Could you check a few things on this model? Use its own coordinates, in mm. Face numbers are marked on the shaded views. A direction names the side the tool comes from. Give positions to 0.01 mm unless a question says otherwise; leave off trailing zeros. Write each loop counter-clockwise with the first axis right and the second up, starting at its lowest first coordinate (ties: lowest second). Pieces come first, ordered by that corner, then holes. Notation, with made-up numbers: M -38.75,-16.75 L -8.75,-16.75 A15 cw -8.75,1.25 Z; hole C -14,89.5 d2. An arc over 180 degrees is marked long. Answer as a JSON object with one key per item and string values. Group by question number.
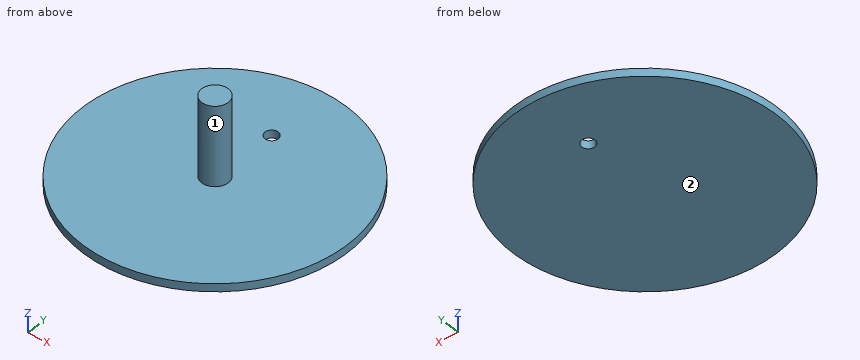
```python
from build123d import *

# Parameters (mm, degrees)
SKETCH_1_R          = 50
EXTRUDE_1_DEPTH     = 3
SKETCH_2_R          = 5
EXTRUDE_2_DEPTH     = 30
SKETCH_3_R          = 2.5
CUT_EXTRUDE_1_DEPTH = 77.811457479


with BuildPart() as part:
    # Эскиз1 → Бобышка-Вытянуть1 (new body)
    with BuildSketch(Plane.XY):
        Circle(SKETCH_1_R)
    extrude(amount=EXTRUDE_1_DEPTH)

    # Эскиз2 → Бобышка-Вытянуть2 (add)
    with BuildSketch(Plane.XY.offset(3)):
        Circle(SKETCH_2_R)
    extrude(amount=EXTRUDE_2_DEPTH)

    # Эскиз3 → Вырез-Вытянуть1 (cut, through all)
    with BuildSketch(Plane.XY.offset(3)):
        with Locations((0, 25)):
            Circle(SKETCH_3_R)
    extrude(amount=-CUT_EXTRUDE_1_DEPTH, mode=Mode.SUBTRACT)


solid = part.part
```
1) Please list where these lines run through material, in increasing order: line 1 along Y through (x, z) = (0, 2); line 2 along Z through (x, y) = (-18.5, -9.5); line 3 along X through (y, z) = (-4, 21.5). Write a range as from..to.
2) I'm going to push flat-ended pins straight in: pin 1 (10 mm diameter, centred on x = 39.5, y = 3.5, fed in from +Z); pin 2 (3 mm diameter, centred on x = 0, y = 25, fed in from -Z); pin 3 (1 mm diameter, centred on x = -19, y = 22, fed in from -Z); pin 4 (4 mm diameter, centred on x = 2, z = 11, fed in from -Y). Where does each tip first touch, or does it pass through?
3) If we section it at A-A, the plane x = 0: List the corners of the cut face in (y, z) for me, plus the area to 3 significant figures.
4) If we section it at D-D, the plane z = 5.5: List the corners of the cut face in (x, y) for me, plus the area to 3 significant figures.
5) For the marked faces 1 and 2, which set-ups out of +Z, -Z, +X, -X, +Y, -Y let a thin tool reach every point of the face, with its end or its side?
6) If we section it at C-C, the plane y = 0: List the corners of the cut face in (x, z) for me.
7) If we section it at B-B, the plane y = 25: List the corners of the cut face in (x, z) for me, plus the area to 3 significant figures.
Taken from the geometry:
{
 "1": {"line 1": "-50..22.5, 27.5..50", "line 2": "0..3", "line 3": "-3..3"},
 "2": {"pin 1": "z = 3", "pin 2": "through", "pin 3": "z = 0", "pin 4": "y = -5"},
 "3": {"outline": "M -50,0 L 22.5,0 L 22.5,3 L 5,3 L 5,33 L -5,33 L -5,3 L -50,3 Z; M 27.5,0 L 50,0 L 50,3 L 27.5,3 Z", "area": "585 mm²"},
 "4": {"outline": "C 0,0 d10", "area": "78.5 mm²"},
 "5": {"face 1": "+Z", "face 2": "-Z, +X, -X, +Y, -Y"},
 "6": {"outline": "M -50,0 L 50,0 L 50,3 L 5,3 L 5,33 L -5,33 L -5,3 L -50,3 Z"},
 "7": {"outline": "M -43.3,0 L -2.5,0 L -2.5,3 L -43.3,3 Z; M 2.5,0 L 43.3,0 L 43.3,3 L 2.5,3 Z", "area": "245 mm²"}
}
